from build123d import *

# Parameters (mm, degrees)
F3_R = 6.35


# Not quite as in the source:
# - a fillet or chamfer that OpenCascade refuses, or shapes differently, is made with other operations: its cross-section is extruded or revolved along the edge and cut away or added


with BuildPart() as f1:
    # F0 (on Front) → F1 (revolve)
    with BuildSketch(Plane.XZ):
        Polygon((-75.2320736647, 15.875), (-75.2320736647, 0), (38.2805263353, 0), (38.2805263353, 6.35), (-71.0156736647, 6.35), (-71.2696736647, 6.35), (-71.2696736647, 15.875), align=None)
    revolve(axis=Axis((-17.1681363136, 0, 20.6502), (1, 0, 0)))

    # F2: fillet of radius 6.35 on 2 edges, made by hand

    # F2_s1 → F2_t2 (revolve, cut)
    with BuildSketch(Plane.XZ):
        with BuildLine():
            ThreePointArc((31.9305263353, 0), (36.4206543959, 1.8598719395), (38.2805263353, 6.35))
            Line((38.2805263353, 6.35), (38.2805263353, 0))
            Line((38.2805263353, 0), (31.9305263353, 0))
        make_face()
    revolve(axis=Axis((38.2805263353, 0, 20.6502), (1, 0, 0)), mode=Mode.SUBTRACT)

    # F2_s3 → F2_t4 (revolve, cut)
    with BuildSketch(Plane.XZ):
        with BuildLine():
            ThreePointArc((-71.2696736647, 9.9909651395), (-72.3526175609, 13.5378821106), (-75.2320736647, 15.875))
            Line((-75.2320736647, 15.875), (-71.2696736647, 15.875))
            Line((-71.2696736647, 15.875), (-71.2696736647, 9.9909651395))
        make_face()
    revolve(axis=Axis((-71.2696736647, 0, 20.6502), (1, 0, 0)), mode=Mode.SUBTRACT)

    # F3
    f3_edges = [f1.edges().sort_by_distance(p)[0] for p in [
        (-75.232074, 0, 41.3004),
    ]]
    fillet(f3_edges, radius=F3_R)


solid = f1.part
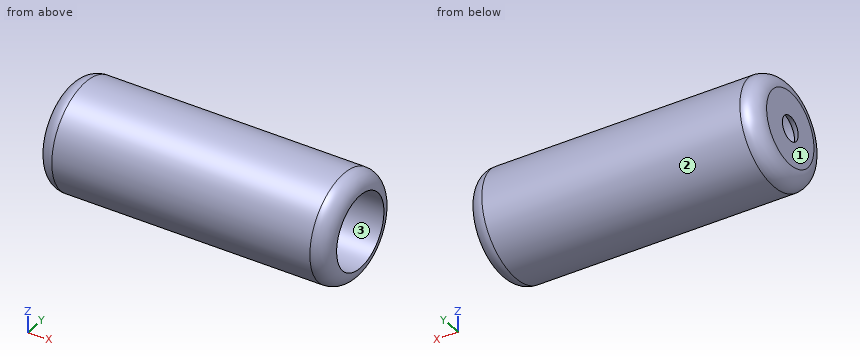
Geometry check sheet. Reference: the model listing, model coordinates, mm. Face numbers are marked on the shaded views. Give positions to 0.01 mm unless a question says otherwise; leave off trailing zeros. Loops run counter-clockwise (first coordinate to the right, second up) from the corner with the lowest first, then second, coordinate; pieces in that order, holes last. Notation, with made-up numbers: M 34,89.25 L 49,89.25 A34 cw 49,128.25 Z; hole C 24.25,-23 d9. An arc over 180 degrees is marked long. Write each question's results on one line, items separated by ' | '.
1) Thickness scan on line 1 (Y direction, x = 27.5, z = 20); line 2 (Z direction, x = -60, y = 9); line 3 (Y direction, x = 24, z = 15.5). Record the ranges inside material, lowest first.
Answers follow:
line 1: -20.64 to -14.29, 14.29 to 20.64 | line 2: 2.06 to 9.54, 31.76 to 39.24 | line 3: -20 to -13.34, 13.34 to 20
2) Release check for a two-part mould opening along Z. For the marked faces 1, 2 and 3 record: +Z half, -Z half, draft (parallel to the pull), parting line (faces both ways), or undercut.
Answers follow:
face 1: draft | face 2: parting line | face 3: undercut
3) Section check B-B, the plane x = -25. Record the boundary of the cut face in (y, z).
Answers follow:
outline: C 0,20.65 d41.3; hole C 0,20.65 d28.6
4) Section check A-A, the plane y = 0. Record the boundary of the cut face in (x, z) (3 decimals).
Answers follow:
outline: M -75.232,6.35 A6.35 ccw -68.882,0 L 31.931,0 A6.35 ccw 38.281,6.35 L -71.27,6.35 L -71.27,9.991 A6.35 ccw -75.232,15.875 Z; M -75.232,25.425 A6.35 ccw -71.27,31.309 L -71.27,34.95 L 38.281,34.95 A6.35 ccw 31.931,41.3 L -68.882,41.3 A6.35 ccw -75.232,34.95 Z
5) Gauge pin test, flat ends, axial feed: pin 1 (1 mm diameter, centred on y = 15.5, z = 17, fed in from -X); pin 2 (4 mm diameter, centred on x = -35.5, y = -7.5, fed in from +Z); pin 3 (4 mm diameter, centred on x = -27.5, z = 31.5, fed in from -Y). Record the tip position at first contact, or that the pin passes through.
Answers follow:
pin 1: x = -75.13 | pin 2: z = 40.55 | pin 3: y = -18.66
